Geometry: final body of the model. Coordinates: model frame, mm. Face numbers are marked on the shaded views. A direction names the side the tool comes from. Coordinates: 2 decimals unless noted, no trailing zeros. Answer as a JSON object with one key per item and string values. Group by question number.
Item 1: Line query: line 1 along X through (y, z) = (2.4, 0); line 2 along Y through (x, z) = (-0.5, 8.5); line 3 along Z through (x, y) = (-1, 1.75). Output: solid intervals per line, ascending. Write a range as from..to.
Item 2: Set-up query: the marked faces 4, 5 and 6. Return all of +Z, -Z, +X, -X, +Y, -Y with unobstructed straight access to the full face (end or side cutting, diameter ignored); none if empty.
Item 3: Section A-A on y = -2.25. State how many separate pieces and enclosed holes the cut face has, and give its area (3 significant figures).
Item 4: Mould query, pull axis X, two halves, no side actions, for the marked faces 1, 2 and 3. Classes: pulls with the +X half, pulls with the -X half, needs draft (parallel to the pull), parting line crosses it, or undercut.
Item 5: First-contact query: pin 1 Ø4.5 at (x, y) = (-11, -4.5) entering from -Z; pin 2 Ø1.2 at (y, z) = (-4.5, 11) entering from -X; pin 3 Ø4 at (y, z) = (-10, 2) entering from -X; pin 4 Ø8 at (y, z) = (-15.5, -10) entering from -X. Flat tips, straight axial feed; report the tip coordinate or a pass-through.
```python
from build123d import *
from build123d.topology import SkipClean

# Parameters (mm, degrees)
BOSS_EXTRUDE2_DEPTH     = 25
BOSS_EXTRUDE2_2_DEPTH   = 25
BOSS_EXTRUDE2_3_DEPTH   = 25
BOSS_EXTRUDE2_4_DEPTH   = 25
BOSS_EXTRUDE3_START     = 3
SKETCH1_4_R             = 13
SKETCH1_4_R_2           = 1.5
SKETCH1_4_R_3           = 3.5
BOSS_EXTRUDE3_DEPTH     = 3
SKETCH1_7_R             = 1.5
CUT_EXTRUDE2_DEPTH      = 3
BOSS_EXTRUDE4_START     = -10
BOSS_EXTRUDE4_DEPTH     = 15
BOSS_EXTRUDE6_DEPTH     = 25
BOSS_EXTRUDE7_DEPTH     = 15
CUT_EXTRUDE1_DEPTH      = 47.121315646
CUT_EXTRUDE1_DEPTH_BACK = 47.121315646


with BuildPart() as part:
    # Sketch1 → Boss-Extrude2 (new body)
    with BuildSketch(Plane(origin=(0, 0, 0), x_dir=(1, 0, 0), z_dir=(0, 1, 0))):
        with BuildLine():
            ThreePointArc((2.781074433, 5.875), (4.596194078, 4.596194078), (5.875, 2.781074433))
            ThreePointArc((5.875, 2.781074433), (7.29221482, 2.985734499), (8.642857143, 2.510183342))
            ThreePointArc((8.642857143, 2.510183342), (6.363961031, 6.363961031), (2.510183342, 8.642857143))
            ThreePointArc((2.510183342, 8.642857143), (2.985734499, 7.29221482), (2.781074433, 5.875))
        make_face()
    extrude(amount=-BOSS_EXTRUDE2_DEPTH)


with BuildPart() as body_2:
    # Sketch1 → Boss-Extrude2 2 (new body)
    with BuildSketch(Plane(origin=(0, 0, 0), x_dir=(1, 0, 0), z_dir=(0, 1, 0))):
        with BuildLine():
            ThreePointArc((8.642857143, -2.510183342), (7.29221482, -2.985734499), (5.875, -2.781074433))
            ThreePointArc((5.875, -2.781074433), (4.596194078, -4.596194078), (2.781074433, -5.875))
            ThreePointArc((2.781074433, -5.875), (2.985734499, -7.29221482), (2.510183342, -8.642857143))
            ThreePointArc((2.510183342, -8.642857143), (6.363961031, -6.363961031), (8.642857143, -2.510183342))
        make_face()
    extrude(amount=-BOSS_EXTRUDE2_2_DEPTH)


    add(part.part)  # Boss-Extrude3 merges part


with BuildPart() as body_3:
    # Sketch1 → Boss-Extrude2 3 (new body)
    with BuildSketch(Plane(origin=(0, 0, 0), x_dir=(1, 0, 0), z_dir=(0, 1, 0))):
        with BuildLine():
            ThreePointArc((-5.875, 2.781074433), (-4.596194078, 4.596194078), (-2.781074433, 5.875))
            ThreePointArc((-2.781074433, 5.875), (-2.985734499, 7.29221482), (-2.510183342, 8.642857143))
            ThreePointArc((-2.510183342, 8.642857143), (-6.363961031, 6.363961031), (-8.642857143, 2.510183342))
            ThreePointArc((-8.642857143, 2.510183342), (-7.29221482, 2.985734499), (-5.875, 2.781074433))
        make_face()
    extrude(amount=-BOSS_EXTRUDE2_3_DEPTH)


with BuildPart() as body_4:
    # Sketch1 → Boss-Extrude2 4 (new body)
    with BuildSketch(Plane(origin=(0, 0, 0), x_dir=(1, 0, 0), z_dir=(0, 1, 0))):
        with BuildLine():
            ThreePointArc((-2.510183342, -8.642857143), (-2.985734499, -7.29221482), (-2.781074433, -5.875))
            ThreePointArc((-2.781074433, -5.875), (-4.596194078, -4.596194078), (-5.875, -2.781074433))
            ThreePointArc((-5.875, -2.781074433), (-7.29221482, -2.985734499), (-8.642857143, -2.510183342))
            ThreePointArc((-8.642857143, -2.510183342), (-6.363961031, -6.363961031), (-2.510183342, -8.642857143))
        make_face()
    extrude(amount=-BOSS_EXTRUDE2_4_DEPTH)


with BuildPart() as body_2_1:
    add(body_2.part)

    add(body_3.part)  # Boss-Extrude3 merges body 3
    # Sketch1<4> → Boss-Extrude3 (add)
    with BuildSketch(Plane(origin=(0, 0, 0), x_dir=(1, 0, 0), z_dir=(0, 1, 0)).offset(BOSS_EXTRUDE3_START)):
        with Locations(Location((0, 0, 0), (0, 0, 270))):
            Circle(SKETCH1_4_R)
        with Locations(Location((7, 0, 0), (0, 0, 270))):
            Circle(SKETCH1_4_R_2, mode=Mode.SUBTRACT)
        with Locations((0, -7)):
            Circle(SKETCH1_4_R_2, mode=Mode.SUBTRACT)
        with Locations((-7, 0)):
            Circle(SKETCH1_4_R_2, mode=Mode.SUBTRACT)
        with Locations(Location((0, 0, 0), (0, 0, 270))):
            Circle(SKETCH1_4_R_3, mode=Mode.SUBTRACT)
        with BuildLine():
            ThreePointArc((1.355261854, 6.357142857), (0, 5.5), (-1.355261854, 6.357142857))
            ThreePointArc((-1.355261854, 6.357142857), (0, 6.5), (1.355261854, 6.357142857))
        make_face(mode=Mode.SUBTRACT)
    extrude(amount=-BOSS_EXTRUDE3_DEPTH)

    # Sketch1<7> → Cut-Extrude2 (cut)
    with BuildSketch(Plane(origin=(0, 0, 0), x_dir=(1, 0, 0), z_dir=(0, 1, 0))):
        with Locations(Location((0, 7, 0), (0, 0, 270))):
            Circle(SKETCH1_7_R)
    extrude(amount=CUT_EXTRUDE2_DEPTH, mode=Mode.SUBTRACT)

    # Sketch1<6> → Boss-Extrude4 (add)
    with BuildSketch(Plane(origin=(0, 0, 0), x_dir=(1, 0, 0), z_dir=(0, 1, 0)).offset(BOSS_EXTRUDE4_START)):
        with BuildLine():
            ThreePointArc((5.875, -2.781074433), (7.29221482, -2.985734499), (8.642857143, -2.510183342))
            ThreePointArc((8.642857143, -2.510183342), (9, 0), (8.642857143, 2.510183342))
            ThreePointArc((8.642857143, 2.510183342), (7.29221482, 2.985734499), (5.875, 2.781074433))
            ThreePointArc((5.875, 2.781074433), (6.5, 0), (5.875, -2.781074433))
        make_face()
        with BuildLine():
            ThreePointArc((2.781074433, 5.875), (2.985734499, 7.29221482), (2.510183342, 8.642857143))
            ThreePointArc((2.510183342, 8.642857143), (0, 9), (-2.510183342, 8.642857143))
            ThreePointArc((-2.510183342, 8.642857143), (-2.985734499, 7.29221482), (-2.781074433, 5.875))
            ThreePointArc((-2.781074433, 5.875), (0, 6.5), (2.781074433, 5.875))
        make_face()
        with BuildLine():
            ThreePointArc((2.510183342, -8.642857143), (2.985734499, -7.29221482), (2.781074433, -5.875))
            ThreePointArc((2.781074433, -5.875), (0, -6.5), (-2.781074433, -5.875))
            ThreePointArc((-2.781074433, -5.875), (-2.985734499, -7.29221482), (-2.510183342, -8.642857143))
            ThreePointArc((-2.510183342, -8.642857143), (0, -9), (2.510183342, -8.642857143))
        make_face()
        with BuildLine():
            ThreePointArc((-5.875, 2.781074433), (-7.29221482, 2.985734499), (-8.642857143, 2.510183342))
            ThreePointArc((-8.642857143, 2.510183342), (-9, 0), (-8.642857143, -2.510183342))
            ThreePointArc((-8.642857143, -2.510183342), (-7.29221482, -2.985734499), (-5.875, -2.781074433))
            ThreePointArc((-5.875, -2.781074433), (-6.5, 0), (-5.875, 2.781074433))
        make_face()
    extrude(amount=-BOSS_EXTRUDE4_DEPTH)


    with SkipClean():  # the faces are left unmerged after this step: merging them gives an invalid solid
        add(body_4.part)  # Boss-Extrude6 merges body 4
        # Sketch3 → Boss-Extrude6 (add)
        with BuildSketch(Plane.XZ):
            with BuildLine():
                Line((-8.485281374, -3), (-12.649110641, -3))
                ThreePointArc((-12.649110641, -3), (-9.192388155, -9.192388155), (-3, -12.649110641))
                Line((-3, -12.649110641), (-3, -8.485281374))
                ThreePointArc((-3, -8.485281374), (-6.363961031, -6.363961031), (-8.485281374, -3))
            make_face()
            with BuildLine():
                ThreePointArc((3, -12.649110641), (9.192388155, -9.192388155), (12.649110641, -3))
                Line((12.649110641, -3), (8.485281374, -3))
                ThreePointArc((8.485281374, -3), (6.363961031, -6.363961031), (3, -8.485281374))
                Line((3, -8.485281374), (3, -12.649110641))
            make_face()
            with BuildLine():
                ThreePointArc((12.649110641, 3), (9.192388155, 9.192388155), (3, 12.649110641))
                Line((3, 12.649110641), (3, 8.485281374))
                ThreePointArc((3, 8.485281374), (6.363961031, 6.363961031), (8.485281374, 3))
                Line((8.485281374, 3), (12.649110641, 3))
            make_face()
            with BuildLine():
                Line((-3, 8.485281374), (-3, 12.649110641))
                ThreePointArc((-3, 12.649110641), (-9.192388155, 9.192388155), (-12.649110641, 3))
                Line((-12.649110641, 3), (-8.485281374, 3))
                ThreePointArc((-8.485281374, 3), (-6.363961031, 6.363961031), (-3, 8.485281374))
            make_face()
        extrude(amount=BOSS_EXTRUDE6_DEPTH)

    # Sketch4 → Boss-Extrude7 (add)
    with SkipClean():  # the faces are left unmerged after this step: merging them gives an invalid solid
        with BuildSketch(Plane.XZ.offset(25)):
            with BuildLine():
                Line((3, -12.649110641), (3, -8.485281374))
                ThreePointArc((3, -8.485281374), (0, -9), (-3, -8.485281374))
                Line((-3, -8.485281374), (-3, -12.649110641))
                ThreePointArc((-3, -12.649110641), (0, -13), (3, -12.649110641))
            make_face()
            with BuildLine():
                ThreePointArc((-8.485281374, -3), (-9, 0), (-8.485281374, 3))
                Line((-8.485281374, 3), (-12.649110641, 3))
                ThreePointArc((-12.649110641, 3), (-13, 0), (-12.649110641, -3))
                Line((-12.649110641, -3), (-8.485281374, -3))
            make_face()
            with BuildLine():
                ThreePointArc((8.485281374, 3), (8.870387037, 1.521917809), (9, 0))
                ThreePointArc((9, 0), (8.870387037, -1.521917809), (8.485281374, -3))
                Line((8.485281374, -3), (12.649110641, -3))
                ThreePointArc((12.649110641, -3), (12.911979676, -1.510225425), (13, 0))
                ThreePointArc((13, 0), (12.911979676, 1.510225425), (12.649110641, 3))
                Line((12.649110641, 3), (8.485281374, 3))
            make_face()
            with BuildLine():
                ThreePointArc((-3, 8.485281374), (0, 9), (3, 8.485281374))
                Line((3, 8.485281374), (3, 12.649110641))
                ThreePointArc((3, 12.649110641), (0, 13), (-3, 12.649110641))
                Line((-3, 12.649110641), (-3, 8.485281374))
            make_face()
        extrude(amount=-BOSS_EXTRUDE7_DEPTH)

    # Sketch2 → Cut-Extrude1 (cut, two sides: drawn at the far end of the back side and taken through both)
    with SkipClean():  # the faces are left unmerged after this step: merging them gives an invalid solid
        with BuildSketch(Plane(origin=(20.02081528, 0, -7.292893219), x_dir=(-0.7071067811865485, 0, 0.7071067811865466), z_dir=(-0.7071067811865466, 0, -0.7071067811865485)).offset(-CUT_EXTRUDE1_DEPTH_BACK)):
            with BuildLine():
                Line((16.813708499, -14.5), (16.813708499, -19))
                ThreePointArc((16.813708499, -19), (19.313708499, -21.5), (21.813708499, -19))
                Line((21.813708499, -19), (21.813708499, -14.5))
                ThreePointArc((21.813708499, -14.5), (19.313708499, -12), (16.813708499, -14.5))
            make_face()
        extrude(amount=CUT_EXTRUDE1_DEPTH + CUT_EXTRUDE1_DEPTH_BACK, mode=Mode.SUBTRACT)


solid = body_2_1.part
```
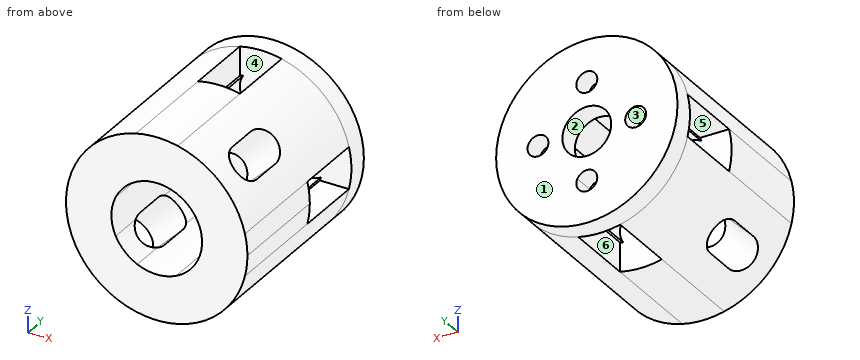
Checks:
{
 "1": {"line 1": "-13..-8.5, -5.5..-3.5, 3.5..5.5, 8.5..13", "line 2": "-25..-10, 0..3", "line 3": "-12.96..-8.12, -5.88..-3.35, 3.35..5.88, 8.12..12.96"},
 "2": {"face 4": "none", "face 5": "-X", "face 6": "-Z"},
 "3": {"separate pieces": "4", "enclosed holes": "0", "area": "242 mm^2"},
 "4": {"face 1": "needs draft", "face 2": "undercut", "face 3": "undercut"},
 "5": {"pin 1": "z = -9.61", "pin 2": "x = -7.8", "pin 3": "x = -13", "pin 4": "x = -11.53"}
}
